Design review of the part built by this model. Coordinates are the model's own, in mm. Face numbers are marked on the shaded views. A direction names the side the tool comes from. Round coordinates to 2 decimals unless told otherwise and drop trailing zeros. Loops run counter-clockwise (first coordinate to the right, second up) from the corner with the lowest first, then second, coordinate; pieces in that order, holes last. Notation, with made-up numbers: (75.25, 12) - (125.25, 12) arc R30 cw to (125.25, 35) - close; hole circle Ø5 at (33, 87.5). An arc over 180 degrees is marked (long way). Return JSON: item names as keys, results as strings. Group by question number.
(1) Wall thickness on L1, parallel to Z at x = -8.25, y = 1; L2, parallel to X at y = -2.75, z = 25.5; L3, parallel to X at y = -2.25, z = 29.5: over which ranges is each line inside the solid? List them lowest first. Write a range as [from, to].
(2) Clearance check with flat-ended pins moving along their axes: pin 1 (7.5 mm diameter, centred on x = 6, z = 57.5, fed in from +Y); pin 2 (1.8 mm diameter, centred on x = -12.5, z = 61, fed in from -Y); pin 3 (8 mm diameter, centred on y = 3, z = 35.5, fed in from -X). State where each tip first meets the part, or that it passes through.
(3) The part is to be moulded in two halves that separate along X. For the marked faces 3, 4 and 5, say which applies: pulls with the +X half, pulls with the -X half, needs draft (parallel to the pull), parting line crosses it, or undercut.
(4) We need section A-A, the plane z = 27.5. Write out the cut boundary in (x, y), and give its area (3 significant figures).
(5) We need section C-C, the plane y = 9.5. Give the number of separate pieces and of enclosed holes in the cut face, and give its area (3 significant figures).
(6) We need section B-B, the plane x = -9.75. Write out the cut boundary in (y, z).
(7) We need section D-D, the plane z = 4. Write out the cut boundary in (x, y).
(8) For the marked faces 1 and 2, list the 3-axis set-ups (+Z, -Z, +X, -X, +Y, -Y) from which the entire face can be reached by the end or side of a thin tool; tool diameter is ignored.
from build123d import *

# Parameters (mm, degrees)
SALIENTE_EXTRUIR1_DEPTH = 82
CROQUIS3_W              = 10
CROQUIS3_H              = 25
SALIENTE_EXTRUIR2_DEPTH = 1.5
CROQUIS4_W              = 18.5
CROQUIS4_H              = 16
SALIENTE_EXTRUIR3_DEPTH = 2
CROQUIS5_R              = 14.5
CORTAR_EXTRUIR1_DEPTH   = 10
CROQUIS9_R              = 0.5
CORTAR_EXTRUIR5_DEPTH   = 10
CORTAR_EXTRUIR6_DEPTH   = 2
CROQUIS11_W             = 10
CROQUIS11_H             = 13
CROQUIS11_W_2           = 18
CROQUIS11_W_3           = 8.121089167
CROQUIS11_H_2           = 20.058238939
CORTAR_EXTRUIR7_DEPTH   = 10
CROQUIS12_W             = 2
CROQUIS12_H             = 13.081043671
CORTAR_EXTRUIR8_DEPTH   = 60
CROQUIS13_W             = 10.5
CROQUIS13_H             = 66
CORTAR_EXTRUIR9_DEPTH   = 12
CROQUIS14_W             = 6
CROQUIS14_H             = 25
SALIENTE_EXTRUIR4_DEPTH = 3
CROQUIS15_R             = 0.5
CORTAR_EXTRUIR10_DEPTH  = 81.950919234


with BuildPart() as part:
    # Croquis2 → Saliente-Extruir1 (new body)
    with BuildSketch(Plane.XY):
        Polygon((-4.596277774, 11.502403514), (-4.596277774, -1.497596486), (9.903722226, -1.497596486), (9.903722226, -4.497596486), (-4.596277774, -4.497596486), (-8.596277774, -4.497596486), (-8.596277774, 11.502403514), align=None)
    extrude(amount=SALIENTE_EXTRUIR1_DEPTH)

    # Croquis3 → Saliente-Extruir2 (add)
    with BuildSketch(Plane(origin=(0, 11.502403514, 0), x_dir=(1, 0, 0), z_dir=(0, 1, 0))):
        with Locations((-9.596277774, -30.5)):
            Rectangle(CROQUIS3_W, CROQUIS3_H)
        with Locations((-9.596277774, -65.5)):
            Rectangle(CROQUIS3_W, CROQUIS3_H)
    extrude(amount=SALIENTE_EXTRUIR2_DEPTH)

    # Croquis4 → Saliente-Extruir3 (add)
    with BuildSketch(Plane(origin=(0, 0, 0), x_dir=(-1, 0, 0), z_dir=(0, 0, -1))):
        with Locations((-0.653722226, 3.502403514)):
            Rectangle(CROQUIS4_W, CROQUIS4_H)
    extrude(amount=SALIENTE_EXTRUIR3_DEPTH)

    # Croquis5 → Cortar-Extruir1 (cut)
    with BuildSketch(Plane(origin=(0, -1.497596486, 0), x_dir=(1, 0, 0), z_dir=(0, 1, 0))):
        with Locations((9.903722226, -82)):
            Circle(CROQUIS5_R)
    extrude(amount=-CORTAR_EXTRUIR1_DEPTH, mode=Mode.SUBTRACT)

    # Croquis9 → Cortar-Extruir5 (cut)
    with BuildSketch(Plane.XZ.offset(-11.502403514)):
        with Locations(Location((-11.596277774, 65.5, 0), (0, 0, 270))):
            Circle(CROQUIS9_R)
        with Locations(Location((-11.596277774, 59.25, 0), (0, 0, 270))):
            Circle(CROQUIS9_R)
        with Locations(Location((-11.596277774, 71.75, 0), (0, 0, 270))):
            Circle(CROQUIS9_R)
    cortar_extruir5 = extrude(amount=-CORTAR_EXTRUIR5_DEPTH, mode=Mode.SUBTRACT)

    # Simetría1: Cortar-Extruir5 across plane
    add(cortar_extruir5.mirror(Plane(origin=(0, 0, 48), x_dir=(1, 0, 0), z_dir=(0, 0, -1))), mode=Mode.SUBTRACT)

    # Croquis10 → Cortar-Extruir6 (cut)
    with BuildSketch(Plane(origin=(0, 0, -2), x_dir=(-1, 0, 0), z_dir=(0, 0, -1))):
        with BuildLine():
            Line((-9.903722226, -2.497596486), (-9.903722226, 11.502403514))
            Line((-9.903722226, 11.502403514), (4.096277774, 11.502403514))
            ThreePointArc((4.096277774, 11.502403514), (-0.00422729, 1.602908577), (-9.903722226, -2.497596486))
        make_face()
    extrude(amount=-CORTAR_EXTRUIR6_DEPTH, mode=Mode.SUBTRACT)

    # Croquis11 → Cortar-Extruir7 (cut)
    with BuildSketch(Plane.ZY.offset(8.596277774)):
        with Locations((48, 5.002403514)):
            Rectangle(CROQUIS11_W, CROQUIS11_H)
        with Locations((9, 5.002403514)):
            Rectangle(CROQUIS11_W_2, CROQUIS11_H)
        with Locations((82.060544584, 1.473284045)):
            Rectangle(CROQUIS11_W_3, CROQUIS11_H_2)
    extrude(amount=-CORTAR_EXTRUIR7_DEPTH, mode=Mode.SUBTRACT)

    # Croquis12 → Cortar-Extruir8 (cut)
    with BuildSketch(Plane.XY.offset(78)):
        with Locations((-6.596277774, 3.961881679)):
            Rectangle(CROQUIS12_W, CROQUIS12_H)
    extrude(amount=-CORTAR_EXTRUIR8_DEPTH, mode=Mode.SUBTRACT)

    # Croquis13 → Cortar-Extruir9 (cut)
    with BuildSketch(Plane.XZ.offset(4.497596486)):
        with Locations((0.653722226, 33)):
            Rectangle(CROQUIS13_W, CROQUIS13_H)
    extrude(amount=-CORTAR_EXTRUIR9_DEPTH, mode=Mode.SUBTRACT)

    # Croquis14 → Saliente-Extruir4 (add)
    with BuildSketch(Plane.XZ.offset(-11.502403514)):
        with Locations((-11.596277774, 65.5)):
            Rectangle(CROQUIS14_W, CROQUIS14_H)
        with Locations((-11.596277774, 30.5)):
            Rectangle(CROQUIS14_W, CROQUIS14_H)
    extrude(amount=SALIENTE_EXTRUIR4_DEPTH)

    # Croquis15 → Cortar-Extruir10 (cut, through all)
    with BuildSketch(Plane(origin=(0, 11.502403514, 0), x_dir=(1, 0, 0), z_dir=(0, 1, 0))):
        with Locations(Location((-11.596277774, -24.25, 0), (0, 0, 90))):
            Circle(CROQUIS15_R)
        with Locations(Location((-11.596277774, -30.5, 0), (0, 0, 90))):
            Circle(CROQUIS15_R)
        with Locations(Location((-11.596277774, -36.75, 0), (0, 0, 90))):
            Circle(CROQUIS15_R)
        with Locations(Location((-11.596277774, -65.5, 0), (0, 0, 270))):
            Circle(CROQUIS15_R)
        with Locations(Location((-11.596277774, -59.25, 0), (0, 0, 270))):
            Circle(CROQUIS15_R)
        with Locations(Location((-11.596277774, -71.75, 0), (0, 0, 270))):
            Circle(CROQUIS15_R)
    extrude(amount=-CORTAR_EXTRUIR10_DEPTH, mode=Mode.SUBTRACT)


solid = part.part
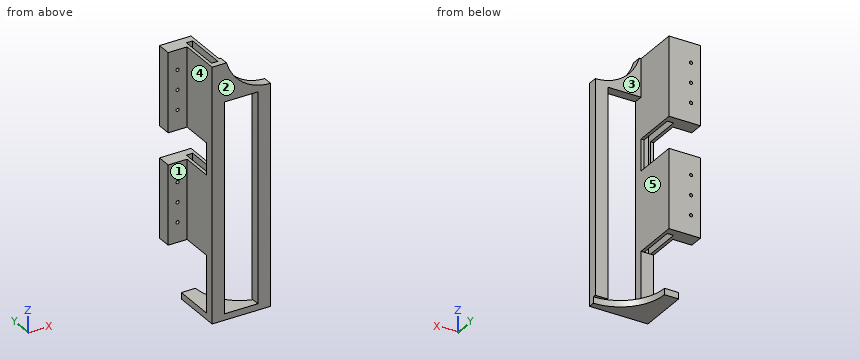
Solutions:
{
 "1": {"L1": "[-2, 0], [18, 43], [53, 78]", "L2": "[-8.6, -4.6], [5.9, 9.9]", "L3": "[-8.6, -7.6], [-5.6, -4.6], [5.9, 9.9]"},
 "2": {"pin 1": "y = -1.5", "pin 2": "y = 8.5", "pin 3": "x = -8.6"},
 "3": {"face 3": "needs draft", "face 4": "pulls with the -X half", "face 5": "undercut"},
 "4": {"outline": "(-14.6, 8.5) - (-8.6, 8.5) - (-8.6, -4.5) - (-4.6, -4.5) - (-4.6, 13) - (-14.6, 13) - close; (5.9, -4.5) - (9.9, -4.5) - (9.9, -1.5) - (5.9, -1.5) - close; hole (-7.6, -2.58) - (-5.6, -2.58) - (-5.6, 10.5) - (-7.6, 10.5) - close", "area": "82.8 mm^2"},
 "5": {"separate pieces": "5", "enclosed holes": "6", "area": "405 mm^2"},
 "6": {"outline": "(8.5, 18) - (13, 18) - (13, 43) - (8.5, 43) - close; (8.5, 53) - (13, 53) - (13, 78) - (8.5, 78) - close"},
 "7": {"outline": "(-8.6, -4.5) - (-4.6, -4.5) - (-4.6, -1.5) - (-8.6, -1.5) - close; (5.9, -4.5) - (9.9, -4.5) - (9.9, -1.5) - (5.9, -1.5) - close"},
 "8": {"face 1": "+Z, -Z, -X, -Y", "face 2": "+Z, -Z, +X, -X, -Y"}
}
